Geometry: final body of the model. Coordinates: model frame, mm. Round coordinates to 2 decimals unless told otherwise and drop trailing zeros. Loops run counter-clockwise (first coordinate to the right, second up) from the corner with the lowest first, then second, coordinate; pieces in that order, holes last. Notation, with made-up numbers: M 66.5,5 L 122.5,5 A11 ccw 122.5,9 Z; hole C 14.5,-22.75 d9. An arc over 180 degrees is marked long. Answer as a JSON object with one key per item and string values.
from build123d import *

# Parameters (mm, degrees)
CROQUIS1_W              = 15
CROQUIS1_H              = 25
SALIENTE_EXTRUIR2_DEPTH = 2
CROQUIS2_R              = 1.5
CORTAR_EXTRUIR1_DEPTH   = 2
CROQUIS3_W              = 26.611189866
CROQUIS3_H              = 39.098747884
CORTAR_EXTRUIR2_DEPTH   = 0.5


with BuildPart() as part:
    # Croquis1 → Saliente-Extruir2 (new body)
    with BuildSketch(Plane(origin=(0, 0, 0), x_dir=(1, 0, 0), z_dir=(0, 1, 0))):
        Rectangle(CROQUIS1_W, CROQUIS1_H)
    extrude(amount=SALIENTE_EXTRUIR2_DEPTH)

    # Croquis2 → Cortar-Extruir1 (cut)
    with BuildSketch(Plane(origin=(0, 2, 0), x_dir=(1, 0, 0), z_dir=(0, 1, 0))):
        with Locations(Location((0, 7.5, 0), (0, 0, 270))):
            Circle(CROQUIS2_R)
        with Locations(Location((0, -7.5, 0), (0, 0, 270))):
            Circle(CROQUIS2_R)
    extrude(amount=-CORTAR_EXTRUIR1_DEPTH, mode=Mode.SUBTRACT)

    # Croquis3 → Cortar-Extruir2 (cut)
    with BuildSketch(Plane(origin=(0, 2, 0), x_dir=(1, 0, 0), z_dir=(0, 1, 0))):
        Rectangle(CROQUIS3_W, CROQUIS3_H)
    extrude(amount=-CORTAR_EXTRUIR2_DEPTH, mode=Mode.SUBTRACT)


solid = part.part
1) Section query C-C (z = -7.5). Return the cut outline in (x, y).
Results:
{"outline": "M -7.5,0 L -1.5,0 L -1.5,1.5 L -7.5,1.5 Z; M 1.5,0 L 7.5,0 L 7.5,1.5 L 1.5,1.5 Z"}
2) Ray query, line 1 (X direction, y = 1.15, z = -7.5); line 2 (X direction, y = 0.5, z = 6.5). Return the intervals inside material, ascending.
Results:
{"line 1": "-7.5 to -1.5, 1.5 to 7.5", "line 2": "-7.5 to -1.12, 1.12 to 7.5"}
3) Section query B-B (y = 1.1). Return the cut outline in (x, z).
Results:
{"outline": "M -7.5,-12.5 L 7.5,-12.5 L 7.5,12.5 L -7.5,12.5 Z; hole C 0,-7.5 d3; hole C 0,7.5 d3"}
4) Section query A-A (x = 0). Return the cut outline in (y, z), and give its area (3 significant figures).
Results:
{"outline": "M 0,-12.5 L 1.5,-12.5 L 1.5,-9 L 0,-9 Z; M 0,-6 L 1.5,-6 L 1.5,6 L 0,6 Z; M 0,9 L 1.5,9 L 1.5,12.5 L 0,12.5 Z", "area": "28.5 mm2"}
5) Section query D-D (z = 7.25). Return the cut outline in (x, y), and give its area (3 significant figures).
Results:
{"outline": "M -7.5,0 L -1.48,0 L -1.48,1.5 L -7.5,1.5 Z; M 1.48,0 L 7.5,0 L 7.5,1.5 L 1.48,1.5 Z", "area": "18.1 mm2"}
6) Pull-direction query (Z, two-part tool) for faces 1 (the cylindrical face through (0, 1, -9)), 2 (the flat face through (0, 1, 12.5)), 3 (the flat face through (-7.5, 1, 0)); classes: +Z half, -Z half, draft (parallel to the pull), parting line (faces both ways), or undercut.
Results:
{"face 1": "undercut", "face 2": "+Z half", "face 3": "draft"}
